Verification items for the finished model (mm, model axes). Face numbers are marked on the shaded views. Round coordinates to 2 decimals unless told otherwise and drop trailing zeros. Loops run counter-clockwise (first coordinate to the right, second up) from the corner with the lowest first, then second, coordinate; pieces in that order, holes last. Notation, with made-up numbers: (-5, 51.25) - (37, 51.25) arc R27 cw to (37, 89.25) - close; hole circle Ø6 at (47.25, 34.25). An arc over 180 degrees is marked (long way). Use CSV: the item, a comma, the result in double quotes.
```python
from build123d import *

# Parameters (mm, degrees)
F0_W     = 76.2
F0_H     = 57.15
F1_DEPTH = 3.175
F2_W     = 72.280051
F2_H     = 53.808485
F3_DEPTH = 6.35


with BuildPart() as f1:
    # F0 (on Top) → F1 (new body, symmetric)
    with BuildSketch(Plane.XY):
        with Locations((9.986312, -6.360359)):
            Rectangle(F0_W, F0_H)
    extrude(amount=F1_DEPTH, both=True)

    # F2 (on face) → F3 (cut, through all)
    with BuildSketch(Plane.XY.offset(3.175)):
        with Locations((9.73773, -6.424894)):
            Rectangle(F2_W, F2_H)
    extrude(amount=-F3_DEPTH, mode=Mode.SUBTRACT)


solid = f1.part
```
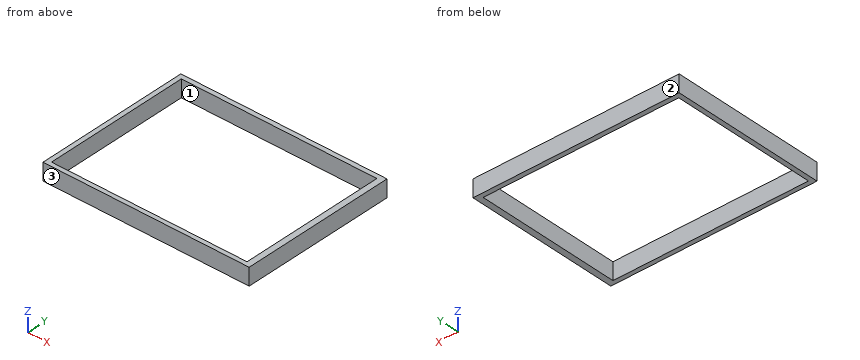
1) Cross-section at A-A, the plane x = 2. Record the cut outline in (y, z) (3 decimals).
Returned:
outline,"(-34.935, -3.175) - (-33.329, -3.175) - (-33.329, 3.175) - (-34.935, 3.175) - close; (20.479, -3.175) - (22.215, -3.175) - (22.215, 3.175) - (20.479, 3.175) - close"
2) Cross-section at B-B, the plane y = 1.5. Record the cut outline in (x, z) (3 decimals).
Returned:
outline,"(-28.114, -3.175) - (-26.402, -3.175) - (-26.402, 3.175) - (-28.114, 3.175) - close; (45.878, -3.175) - (48.086, -3.175) - (48.086, 3.175) - (45.878, 3.175) - close"
3) Cross-section at C-C, the plane z = -0.25. Record the cut outline in (x, y).
Returned:
outline,"(-28.11, -34.94) - (48.09, -34.94) - (48.09, 22.21) - (-28.11, 22.21) - close; hole (-26.4, -33.33) - (45.88, -33.33) - (45.88, 20.48) - (-26.4, 20.48) - close"
4) Mould release check, pull along Y, two halves, no side actions. Record for the marked faces 1, 2 and 3: +Y half, -Y half, draft (parallel to the pull), parting line (faces both ways), or undercut.
Returned:
face 1,"undercut"
face 2,"+Y half"
face 3,"-Y half"
5) Thickness scan on probe 1 along X at (y, z) = (9.5, 1.25); probe 2 along Y at (x, z) = (35, -2.25). Record the ranges inside material, lowest first. Write a range as [from, to].
Returned:
probe 1,"x = [-28.11, -26.4], [45.88, 48.09]"
probe 2,"y = [-34.94, -33.33], [20.48, 22.21]"
